```python
from build123d import *

# Parameters (mm, degrees)
F1_DEPTH      = 20
F4_DEPTH      = 7.0720678119
F4_DEPTH_BACK = 7.0720678119
F8_R          = 0.2
F9_T          = -1


# Not quite as in the source:
# - the program builds the solid bodies; features that only make, move or delete a surface that nothing else refers to are left out


with BuildPart() as f1:
    # F0 (on Right) → F1 (new body)
    with BuildSketch(Plane.YZ):
        Polygon((7.0710678119, 0), (0, 7.0710678119), (-7.0710678119, 0), (0, -7.0710678119), align=None)
    extrude(amount=F1_DEPTH)

    # F3 (on 3pt) → F4 (cut, two sides)
    with BuildSketch(Plane(origin=(0, 0, 0), x_dir=(-1, 0, 0), z_dir=(0, 1, 0))) as f4_sk:
        Polygon((0.2828427125, 7.0710678119), (-7.0710678119, 14.4249783362), (-14.4249783362, 7.0710678119), (-7.0710678119, -0.2828427125), align=None)
    extrude(amount=-F4_DEPTH, mode=Mode.SUBTRACT)
    extrude(f4_sk.sketch, amount=F4_DEPTH_BACK, mode=Mode.SUBTRACT)

    # F7: F1 across face


with BuildPart() as f1_1:
    add(f1.part)
    add(f1.part.mirror(Plane(origin=(0, 0, -0.0055104131), x_dir=(0, 1, 0), z_dir=(-1, 0, 0))))

    # F8
    f8_edges = [f1_1.edges().sort_by_distance(p)[0] for p in [
        (7.071068, 0, -0.282843),
        (3.394113, -3.676955, 3.394113),
        (3.394113, 3.676955, 3.394113),
        (0, 0, 6.788225),
        (6.929646, -6.929646, -0.141421),
        (6.929646, 6.929646, -0.141421),
        (7.212489, 6.929646, -0.141421),
        (7.212489, -6.929646, -0.141421),
        (10.889444, -3.535534, 3.535534),
        (10.889444, 3.535534, 3.535534),
        (17.212489, 0, 7.071068),
        (13.676955, 7.071068, 0),
        (13.676955, -7.071068, 0),
        (0, -7.071068, 0),
        (-13.676955, -7.071068, 0),
        (-7.212489, -6.929646, -0.141421),
        (-6.929646, -6.929646, -0.141421),
        (-10.889444, -3.535534, 3.535534),
        (-3.394113, -3.676955, 3.394113),
        (-3.394113, 3.676955, 3.394113),
        (-7.071068, 0, -0.282843),
        (-7.212489, 6.929646, -0.141421),
        (-6.929646, 6.929646, -0.141421),
        (-10.889444, 3.535534, 3.535534),
        (-17.212489, 0, 7.071068),
        (-13.676955, 7.071068, 0),
        (0, 7.071068, 0),
        (0, 0, -7.071068),
    ]]
    fillet(f8_edges, radius=F8_R)

    # F9
    f9_openings = [f1_1.faces().sort_by_distance(p)[0] for p in [
        (20, 0, 0),
        (-20, 0, 0),
    ]]
    offset(amount=F9_T, openings=f9_openings)


solid = f1_1.part
```
Design review of the part built by this model. Coordinates are the model's own, in mm. A direction names the side the tool comes from. Give positions to 0.01 mm unless a question says otherwise; leave off trailing zeros. Loops run counter-clockwise (first coordinate to the right, second up) from the corner with the lowest first, then second, coordinate; pieces in that order, holes last. Notation, with made-up numbers: M 73.25,42 L 106.25,42 A28 ccw 106.25,69 Z; hole C 37.5,38.5 d1. An arc over 180 degrees is marked long. Return JSON: item names as keys, results as strings. Group by question number.
Item 1: Insertion check: pin 1 Ø1.5 at (x, y) = (-10, -4.5) entering from -Z; pin 2 Ø3 at (y, z) = (-0.5, -0.5) entering from +X; pin 3 Ø5 at (x, y) = (7, 3) entering from -Z; pin 4 Ø1 at (y, z) = (-4, 4) entering from -X. Each pin has a flat end and moves straight along its axis. Give the tip position at first contact, or say it passes through.
Item 2: Mouldability with a two-part tool opening along Z and no side actions: class faces 4 (the flat face through (-10.012, -0.095, 2.658)), 5 (the flat face through (0.28, -2.868, -2.789)), 6 (the flat face through (0.28, 3.49, -3.58)) as released by +Z, released by -Z, zero draft, split by the parting line, or undercut.
Item 3: We need section A-A (x = 17.5). Give the boundary of the cut face in (y, z).
Item 4: We need section C-C (z = 4.75). Give the number of separate pieces and of enclosed holes in the cut face, and give its area (3 significant figures).
Item 5: Tool access review of faces 1 (the flat face through (-10.5, -0.08, 1.73)), 2 (the flat face through (-4.34, -0.1, 2.45)), 3 (the flat face through (0.075, 3.605, 2.052)): name each direction out of +Z, -Z, +X, -X, +Y, -Y from which nothing blocks a thin tool from reaching the whole face with its end or side.
Item 6: For probe 1 along X at (y, z) = (6, 0.5); probe 2 along X at (y, z) = (-0.25, 3.5); probe 3 along X at (y, z) = (3.5, 0.5), list the stretches that pass through material, from the lowest coordinate up.
Item 7: We need section B-B (z = -4). Give the boundary of the cut face in (x, y), and give its area (3 significant figures).
Output:
{
 "1": {"pin 1": "stops at z = -3.32", "pin 2": "stops at x = 9.77", "pin 3": "stops at z = -6.57", "pin 4": "passes through"},
 "2": {"face 4": "released by +Z", "face 5": "undercut", "face 6": "released by -Z"},
 "3": {"outline": "M -6.93,-0.14 L -0.14,-6.93 A0.2 ccw 0.14,-6.93 L 6.93,-0.14 A0.2 ccw 6.93,0.14 L 0.14,6.93 A0.2 ccw -0.14,6.93 L -6.93,0.14 A0.2 ccw Z; hole M -5.66,0 L 0,-5.66 L 5.66,0 L 0,5.66 Z"},
 "4": {"separate pieces": "3", "enclosed holes": "1", "area": "66.4 mm^2"},
 "5": {"face 1": "-X", "face 2": "+Z, +Y, -Y", "face 3": "none"},
 "6": {"probe 1": "x = -20 to -7.85, -6.29 to 6.29, 7.85 to 20", "probe 2": "x = -12.27 to -10.85, -3.29 to -1.87, 1.87 to 3.29, 10.85 to 12.27", "probe 3": "x = -9.27 to -7.85, -6.29 to -4.87, 4.87 to 6.29, 7.85 to 9.27"},
 "7": {"outline": "M -20,-3.07 L 20,-3.07 L 20,-1.66 L -20,-1.66 Z; M -20,1.66 L 20,1.66 L 20,3.07 L -20,3.07 Z", "area": "113 mm^2"}
}
